Build history of the part. All positions in model axes, mm. A direction names the side the tool comes from. Round coordinates to 2 decimals unless told otherwise and drop trailing zeros. Write each loop counter-clockwise with the first axis right and the second up, starting at its lowest first coordinate (ties: lowest second). Pieces come first, ordered by that corner, then holes.
1) Saw through at D-D (y = -1). Write the cut outline in (x, z), plus the area to 3 significant figures.
2) Saw through at A-A (x = 1.25). Write the cut outline in (y, z), plus the area to 3 significant figures.
3) Saw through at C-C (z = -2). Write the cut outline in (x, y), plus the area to 3 significant figures.
4) Wall check: probe 1 along Z at (x, y) = (1.5, -1.75); probe 2 along Y at (x, z) = (4.25, 6); probe 3 along X at (y, z) = (-9.25, 7.5). Give the ranges that are in metal, low to high.
5) Flat gauge pins, fed straight in: pin 1 (5 mm diameter, centred on x = -5, z = 0.5, fed in from -Y); pin 2 (6.5 mm diameter, centred on x = 1, y = -4, fed in from +Z); pin 3 (2 mm diameter, centred on y = -3, z = -8, fed in from -X); pin 4 (1 mm diameter, centred on x = 3, y = -8, fed in from +Z). Where does each tip first touch, or does it go through?
6) Which spindle directions (+Z, -Z, +X, -X, +Y, -Y) get a long thin tool onto all of the face, cutting with end or side? Do faces 1 (the flat face through (0, -7, -14.056)), 2 (the cylindrical face through (-0.52, -8.967, 11.563)). Say none if no direction does.
7) Saw through at B-B (y = -4.5). Write the cut outline in (x, z), plus the area to 3 significant figures.
from build123d import *

# Parameters (mm, degrees)
F0_W        = 13
F0_H        = 25
F1_DEPTH    = 13.3
F2_T1_DEPTH = 60
F3_R        = 2.3988819555
F4_DEPTH    = 12.2


# Not quite as in the source:
# - a fillet or chamfer that OpenCascade refuses, or shapes differently, is made with other operations: its cross-section is extruded or revolved along the edge and cut away or added
# - a feature names something its author has since deleted; it is built from what else it names


with BuildPart() as f1:
    # F0 (on Front) → F1 (new body)
    with BuildSketch(Plane.XZ):
        with Locations((0, -1.5561378314)):
            Rectangle(F0_W, F0_H)
    extrude(amount=F1_DEPTH)

    # F2: fillet of radius 7 on 4 edges, made by hand

    # F2_s2 → F2_t1 (cut)
    with BuildSketch(Plane.XY.offset(-31.5561378314)):
        with BuildLine():
            ThreePointArc((6.5, -6.3), (4.4497474683, -11.2497474683), (-0.5, -13.3))
            Line((-0.5, -13.3), (6.5, -13.3))
            Line((6.5, -13.3), (6.5, -6.3))
        make_face()
        with BuildLine():
            ThreePointArc((6.5, -7), (4.4497474683, -2.0502525317), (-0.5, 0))
            Line((-0.5, 0), (6.5, 0))
            Line((6.5, 0), (6.5, -7))
        make_face()
        with BuildLine():
            ThreePointArc((-6.5, -7), (-4.4497474683, -2.0502525317), (0.5, 0))
            Line((0.5, 0), (-6.5, 0))
            Line((-6.5, 0), (-6.5, -7))
        make_face()
        with BuildLine():
            ThreePointArc((-6.5, -6.3), (-4.4497474683, -11.2497474683), (0.5, -13.3))
            Line((0.5, -13.3), (-6.5, -13.3))
            Line((-6.5, -13.3), (-6.5, -6.3))
        make_face()
    extrude(amount=F2_T1_DEPTH, mode=Mode.SUBTRACT)

    # F3 (on Top) → F4 (join)
    with BuildSketch(Plane.XY):
        with Locations((0, -6.6247042269)):
            Circle(F3_R)
    extrude(amount=F4_DEPTH)


solid = f1.part
Evaluation:
1. outline: (-3.11, -14.06) - (3.11, -14.06) - (3.11, 10.94) - (-3.11, 10.94) - close
1. area: 155 mm2
2. outline: (-13.08, -14.06) - (-0.22, -14.06) - (-0.22, 10.94) - (-4.58, 10.94) - (-4.58, 12.2) - (-8.67, 12.2) - (-8.67, 10.94) - (-13.08, 10.94) - close
2. area: 327 mm2
3. outline: (-6.49, -6.65) arc R7 ccw to (0, -13.28) arc R7 ccw to (6.49, -6.65) arc R7 ccw to (0, -0.02) arc R7 ccw to start
3. area: 131 mm2
4. probe 1: z = -14.06 to 10.94
4. probe 2: y = -11.44 to -1.86
4. probe 3: x = -5.85 to 5.85
5. pin 1: stops at y = -12.62
5. pin 2: stops at z = 12.2
5. pin 3: stops at x = -5.82
5. pin 4: stops at z = 10.94
6. face 1: -Z, +X, -X, +Y, -Y
6. face 2: +Z
7. outline: (-6.04, -14.06) - (6.04, -14.06) - (6.04, 10.94) - (1.11, 10.94) - (1.11, 12.2) - (-1.11, 12.2) - (-1.11, 10.94) - (-6.04, 10.94) - close
7. area: 305 mm2
